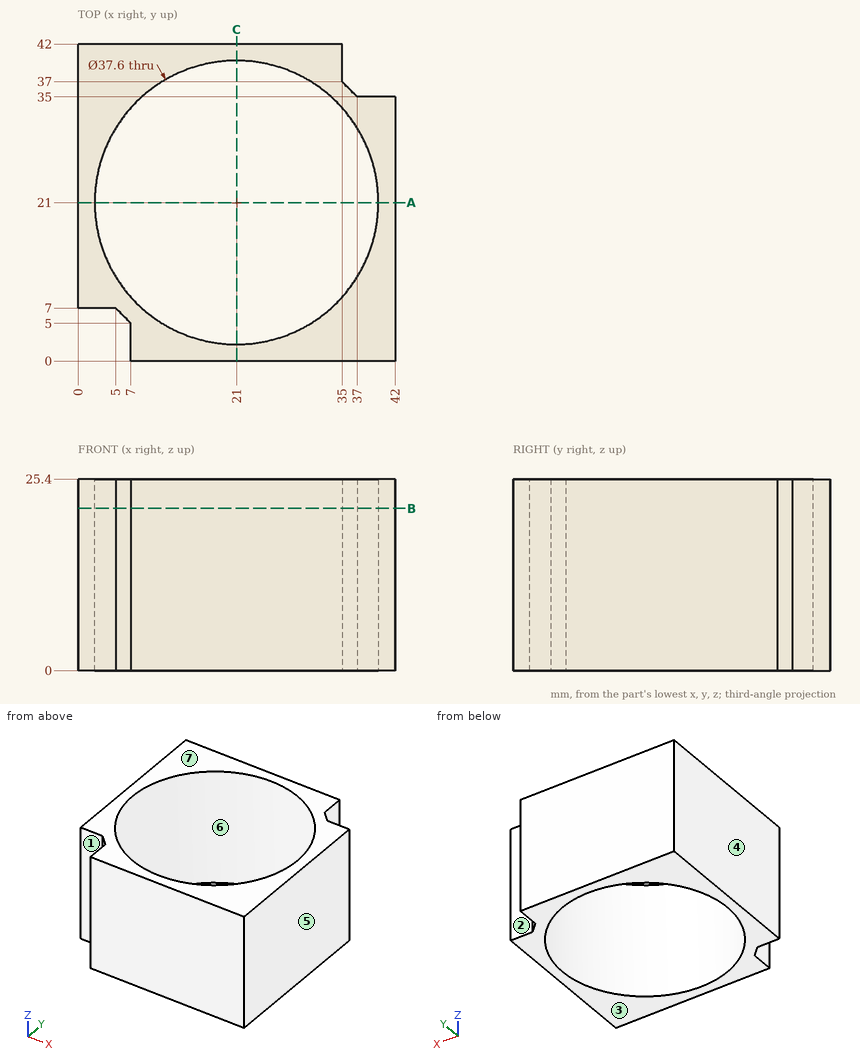
The figure shows three views and two pictorial views of one solid part (mm, origin at its lowest corner). Answer the questions. A direction names the side the tool comes from. Give positions to 0.01 mm unless a question says otherwise; leave off trailing zeros. Write each loop counter-clockwise with the first axis right and the second up, starting at its lowest first coordinate (ties: lowest second). Pieces come first, ordered by that corner, then holes. Notation, with made-up numbers: (-8, -21) - (50, -21) arc R24 cw to (50, 2) - close; hole circle Ø7 at (73.5, 81). An arc over 180 degrees is marked (long way). Use one line per item in the form item = value. Start each with the question number.
1) A tool of negligible diameter and unlimited length cuts with its end or side. For the marked faces 1, 2 and 3, from which of +Z, -Z, +X, -X, +Y, -Y can it reach the whole face along a straight path? Write none if from no direction.
2) Find section B-B on z = 21.5. Determine the outline of the cut face in (x, y).
3) Consider line 1 along Y through (x, z) = (21, 14.75); line 2 along Y through (x, z) = (40, 10.5); line 3 along Y through (x, z) = (27.5, 23.25). Determine where each line is inside the solid, lowest interval first. Write a range as from..to.
4) The mould has two halves that part along X. Classify the marked faces 4, 5, 6 and 7: pulls with the +X half, pulls with the -X half, needs draft (parallel to the pull), parting line crosses it, or undercut.
5) Find section A-A on y = 21. Determine the outline of the cut face in (x, z).
6) Flat-ended cylindrical pins translate along their axes: pin 1 Ø1.5 at (y, z) = (38.5, 17.5) entering from +X; pin 2 Ø5.5 at (x, z) = (40.5, 7.5) entering from +Y; pin 3 Ø5.5 at (x, z) = (1.5, 8) entering from -Y. Find the tip coordinate at first contact, or state that the pin passes through.
Geometry results:
q1.face_1 = +Z, -Z, -X, -Y
q1.face_2 = +Z, -Z, +X, +Y
q1.face_3 = -Z, +X, -X, +Y, -Y
q2.outline = (0, 7) - (5, 7) - (7, 5) - (7, 0) - (42, 0) - (42, 35) - (37, 35) - (35, 37) - (35, 42) - (0, 42) - close; hole circle Ø37.6 at (21, 21)
q3.line_1 = 0..2.2, 39.8..42
q3.line_2 = 0..35
q3.line_3 = 0..3.36, 38.64..42
q4.face_4 = pulls with the -X half
q4.face_5 = pulls with the +X half
q4.face_6 = undercut
q4.face_7 = needs draft
q5.outline = (0, 0) - (2.2, 0) - (2.2, 25.4) - (0, 25.4) - close; (39.8, 0) - (42, 0) - (42, 25.4) - (39.8, 25.4) - close
q6.pin_1 = 35
q6.pin_2 = 35
q6.pin_3 = 7
